The figure shows three views and two pictorial views of one solid part (mm, origin at its lowest corner). Answer the questions. Give positions to 0.01 mm unless a question says otherwise; leave off trailing zeros. Loops run counter-clockwise (first coordinate to the right, second up) from the corner with the lowest first, then second, coordinate; pieces in that order, holes last. Notation, with made-up numbers: M 71,46.5 L 126,46.5 A8 cw 126,53.5 Z; hole C 31.5,56.25 d3. An arc over 180 degrees is marked long. Answer as a JSON object with one key per item and string values. Group by question number.
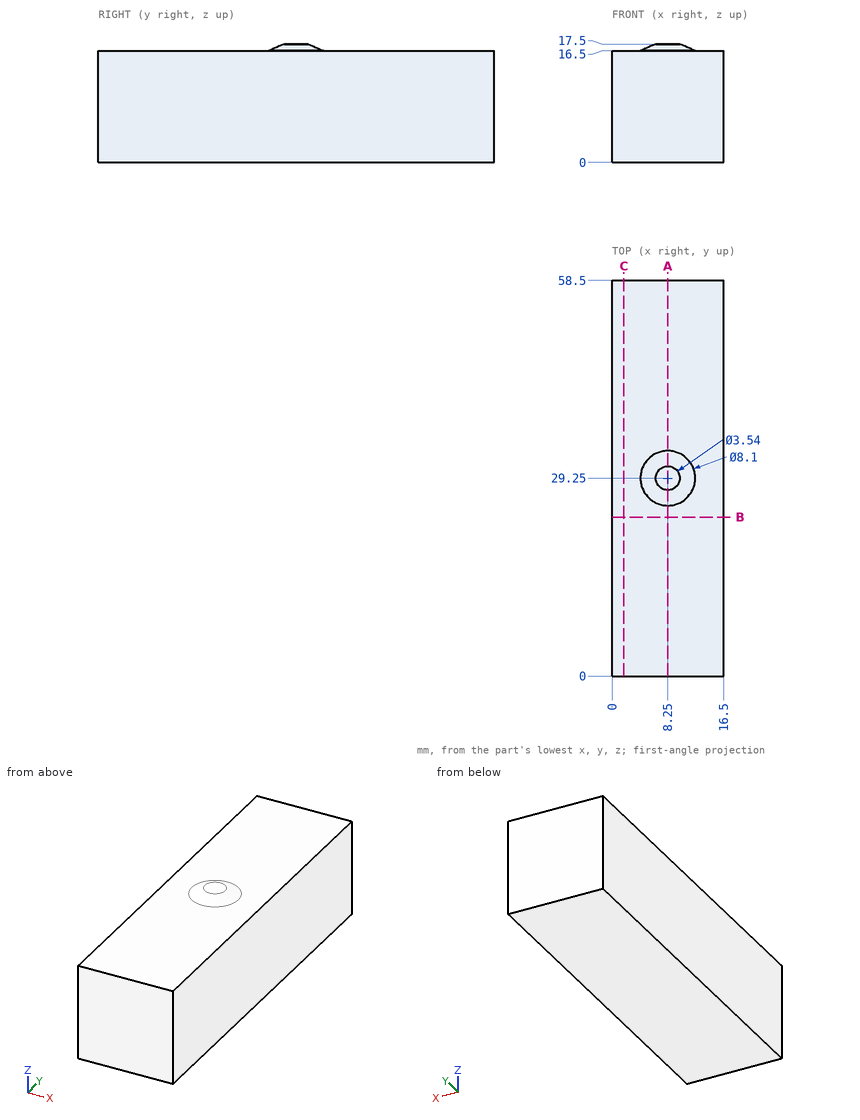
Item 1: A cutting plane is placed at B-B (y = 23.5). Determine the outline of the cut face in (x, z).
Item 2: Given pin 1 Ø6 at (x, y) = (7.5, 12.5) entering from +Z; pin 2 Ø10 at (y, z) = (17, 9) entering from -X, each flat-ended and moving along its own axis, determine where each tip first touches the part or whether it passes through.
Item 3: A cutting plane is placed at A-A (x = 8.25). Determine the outline of the cut face in (y, z).
Item 4: Find the intervals of material crossed by probe 1 along Z at (x, y) = (11, 52), in increasing order. Write a range as [from, to].
Item 5: A cutting plane is placed at C-C (x = 1.75). Determine the outline of the cut face in (y, z), and give its area (3 significant figures).
The answers:
{
 "1": {"outline": "M 0,0 L 16.5,0 L 16.5,16.5 L 0,16.5 Z"},
 "2": {"pin 1": "stops at z = 16.5", "pin 2": "stops at x = 0"},
 "3": {"outline": "M 0,0 L 58.5,0 L 58.5,16.5 L 33.3,16.5 L 31.02,17.5 L 27.48,17.5 L 25.2,16.5 L 0,16.5 Z"},
 "4": {"probe 1": "z = [0, 16.5]"},
 "5": {"outline": "M 0,0 L 58.5,0 L 58.5,16.5 L 0,16.5 Z", "area": "965 mm^2"}
}
